```python
from build123d import *


# Not quite as in the source:
# - a feature names something its author has since deleted; it is built from what else it names


with BuildPart() as f1:
    # F0 (on Front) → F1 (revolve)
    with BuildSketch(Plane.XZ):
        with BuildLine():
            Line((16, -2.4131433771), (7.5, -2.4131433771))
            ThreePointArc((7.5, -2.4131433771), (11.8585412256, 11.5397036981), (0, 20.0868566229))
            Line((0, 20.0868566229), (0, 7.5868566229))
            Line((0, 7.5868566229), (0, -2.4131433771))
            Line((0, -2.4131433771), (0, -17.4131433771))
            Line((0, -17.4131433771), (0, -32.4131433771))
            Line((0, -32.4131433771), (0, -47.4131433771))
            Line((0, -47.4131433771), (0.1347365081, -49.4085997343))
            Line((0.1347365081, -49.4085997343), (0.1347365081, -51.4085997343))
            Line((0.1347365081, -51.4085997343), (27.1347365081, -51.4085997343))
            add(Edge.make_bspline(
                [(20, -49.4085997343), (21.1647466197, -48.7697309267), (24.5158880863, -49.2280358233), (26.0127596557, -50.3029301763), (27.1347365081, -51.4085997343)],
                knots=[0, 0, 0, 0, 0.5171119301, 1, 1, 1, 1], degree=3))
            Line((20, -49.4085997343), (20, -47.4131433771))
            add(Edge.make_bspline(
                [(8, -32.4131433771), (8.1538179197, -34.0022767405), (8.8353543612, -37.329541577), (12.0621827681, -44.6088268089), (17.7756990209, -46.0672005111), (20, -47.4131433771)],
                knots=[0, 0, 0, 0, 0.2858059908, 0.6339622457, 1, 1, 1, 1], degree=3))
            Line((8, -32.4131433771), (8, -17.4131433771))
            add(Edge.make_bspline(
                [(16, -2.4131433771), (14.9209762915, -3.8251770696), (11.0665886907, -6.0967064809), (8.9117025522, -11.4433176222), (8.4714845406, -15.3714061946), (8, -17.4131433771)],
                knots=[0, 0, 0, 0, 0.3360443888, 0.6607253154, 1, 1, 1, 1], degree=3))
        make_face()
    revolve(axis=Axis((0, 0, 13.8368566229), (0, 0, -1)))


solid = f1.part
```
Work out the finished part from the listing and answer in its coordinate system (mm). Coordinates: 2 decimals unless noted, no trailing zeros. Loops run counter-clockwise (first coordinate to the right, second up) from the corner with the lowest first, then second, coordinate; pieces in that order, holes last. Notation, with made-up numbers: (13, -13) - (44, -13) arc R5 ccw to (44, -8) - close; hole circle Ø4 at (89.5, 65.5). An arc over 180 degrees is marked (long way). Use a Markdown table: item, result.
Item 1: The mould has two halves that part along Y. Classify faces 1 (the flat face through (0.4, -0.4, -51.409)), 2 (the cylindrical face through (-1.73, 7.81, -24.81)), 3 (the cylindrical face through (-4.336, 19.524, -48.397)): +Y half, -Y half, draft (parallel to the pull), parting line (faces both ways), or undercut.
Evaluation:
| item | result |
|---|---|
| face 1 | draft |
| face 2 | parting line |
| face 3 | undercut |
Item 2: Find section A-A, the plane y = 10.5. State how many separate pieces and enclosed holes the cut face has, and give its area (3 significant figures).
Evaluation:
| item | result |
|---|---|
| separate pieces | 3 |
| enclosed holes | 0 |
| area | 510 mm2 |
Item 3: Find section B-B, the plane z = -25.5. Determine the outline of the cut face in (x, y).
Evaluation:
| item | result |
|---|---|
| outline | circle Ø16 at (0, 0) |
Item 4: Given pin 1 Ø12 at (x, y) = (20, -11) entering from +Z; pin 2 Ø1.5 at (x, z) = (-2, -41.5) entering from -Y; pin 3 Ø2 at (y, z) = (-9, -2.5) entering from -X, each flat-ended and moving along its own axis, determine where each tip first touches the part or whether it passes through.
Evaluation:
| item | result |
|---|---|
| pin 1 | stops at z = -45.86 |
| pin 2 | stops at y = -11.38 |
| pin 3 | stops at x = -13.85 |
Item 5: Consider probe 1 along Y at (x, z) = (0, -50); probe 2 along Y at (x, z) = (0, -50.2); probe 3 along Z at (x, y) = (-4, -13). Determine where each line is inside the solid, lowest interval first. Write a range as from..to.
Evaluation:
| item | result |
|---|---|
| probe 1 | y = -25.44..-0.13, 0.13..25.44 |
| probe 2 | y = -25.74..-0.13, 0.13..25.74 |
| probe 3 | z = -51.41..-44.19, -4.66..-2.41 |
